```python
from build123d import *

# Parameters (mm, degrees)
SKETCH1_W           = 25.4
SKETCH1_H           = 38.1
BOSS_EXTRUDE1_DEPTH = 2.54
FILLET1_R           = 6.35
CUT_EXTRUDE1_DEPTH  = 0.254


with BuildPart() as part:
    # Sketch1 → Boss-Extrude1 (new body)
    with BuildSketch(Plane.XY):
        Rectangle(SKETCH1_W, SKETCH1_H)
    extrude(amount=BOSS_EXTRUDE1_DEPTH)

    # Fillet1
    fillet1_edges = [part.edges().sort_by_distance(p)[0] for p in [
        (12.7, -19.05, 1.27),
        (-12.7, -19.05, 1.27),
        (-12.7, 19.05, 1.27),
        (12.7, 19.05, 1.27),
    ]]
    fillet(fillet1_edges, radius=FILLET1_R)

    # Sketch2 → Cut-Extrude1 (cut)
    with BuildSketch(Plane.XY.offset(2.54)):
        with BuildLine():
            Line((-6.35, -19.05), (6.35, -19.05))
            ThreePointArc((6.35, -19.05), (10.840128061, -17.190128061), (12.7, -12.7))
            Line((12.7, -12.7), (12.7, 12.7))
            ThreePointArc((12.7, 12.7), (10.840128061, 17.190128061), (6.35, 19.05))
            Line((6.35, 19.05), (-6.35, 19.05))
            ThreePointArc((-6.35, 19.05), (-10.840128061, 17.190128061), (-12.7, 12.7))
            Line((-12.7, 12.7), (-12.7, -12.7))
            ThreePointArc((-12.7, -12.7), (-10.840128061, -17.190128061), (-6.35, -19.05))
        make_face()
        with BuildLine():
            Line((-11.43, 12.7), (-11.43, -12.7))
            ThreePointArc((-11.43, -12.7), (-9.942102448, -16.292102448), (-6.35, -17.78))
            Line((-6.35, -17.78), (6.35, -17.78))
            ThreePointArc((6.35, -17.78), (9.942102448, -16.292102448), (11.43, -12.7))
            Line((11.43, -12.7), (11.43, 12.7))
            ThreePointArc((11.43, 12.7), (9.942102448, 16.292102448), (6.35, 17.78))
            Line((6.35, 17.78), (-6.35, 17.78))
            ThreePointArc((-6.35, 17.78), (-9.942102448, 16.292102448), (-11.43, 12.7))
        make_face(mode=Mode.SUBTRACT)
    extrude(amount=-CUT_EXTRUDE1_DEPTH, mode=Mode.SUBTRACT)


solid = part.part
```
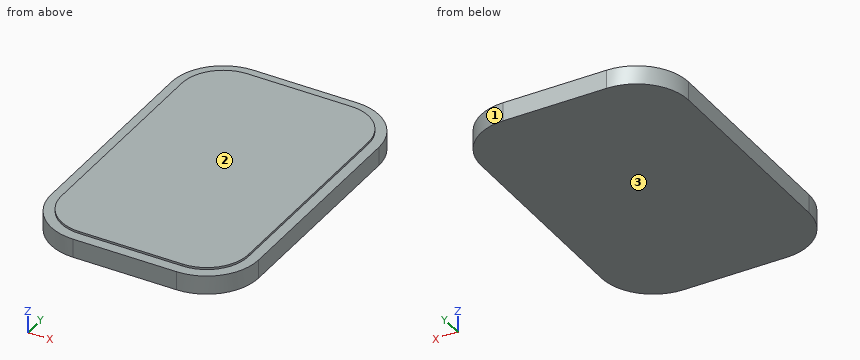
Can you work these out from the model? Positions are in its coordinate system, mm. Face numbers are marked on the shaded views. Give positions to 0.01 mm unless a question says otherwise; leave off trailing zeros. Order: outer loops, then holes, each group sorted by start corner. A loop starts at its lowest first (then second) coordinate and runs counter-clockwise, first axis right, second up. Notation, with made-up numbers: M 12,-20 L 22,-20 A24 cw 22,8 Z; hole C 53.5,-12.75 d3. An arc over 180 degrees is marked long. Write item = value, one per line. Start each with the question number.
Q1. I need wall thicknesses on probe 1 along Z at (x, y) = (11.5, 6); probe 2 along X at (y, z) = (-12.5, 2.4); probe 3 along Y at (x, z) = (-9.5, 0.3). Which ranges of each line are inside material? Lowest first, please. Write a range as [from, to].
Q2. We'd pull the mould along Z, two halves only. Please class the marked faces 1, 2 and 3: pulls with the +Z half, pulls with the -Z half, needs draft (parallel to the pull), parting line crosses it, or undercut.
Q3. Will this pin go through, and if not, where does the flat tip stop? pin 1 Ø1 at (x, z) = (-10, 0.5) entering from -Y.
Q4. Suppose I cut it at B-B (y = -14). Write out the boundary of the cut face in (x, z), plus the area to 3 significant figures.
Q5. Suppose I cut it at A-A (z = 1.35). Write out the boundary of the cut face in (x, y), plus the area to 3 significant figures.
Check result:
q1.probe_1 = [0, 2.29]
q1.probe_2 = [-11.43, 11.43]
q1.probe_3 = [-18.21, 18.21]
q2.face_1 = needs draft
q2.face_2 = pulls with the +Z half
q2.face_3 = pulls with the -Z half
q3.pin_1 = -18.21
q4.outline = M -12.57,0 L 12.57,0 L 12.57,2.29 L 11.26,2.29 L 11.26,2.54 L -11.26,2.54 L -11.26,2.29 L -12.57,2.29 Z
q4.area = 63.2 mm2
q5.outline = M -12.7,-12.7 A6.35 ccw -6.35,-19.05 L 6.35,-19.05 A6.35 ccw 12.7,-12.7 L 12.7,12.7 A6.35 ccw 6.35,19.05 L -6.35,19.05 A6.35 ccw -12.7,12.7 Z
q5.area = 933 mm2
